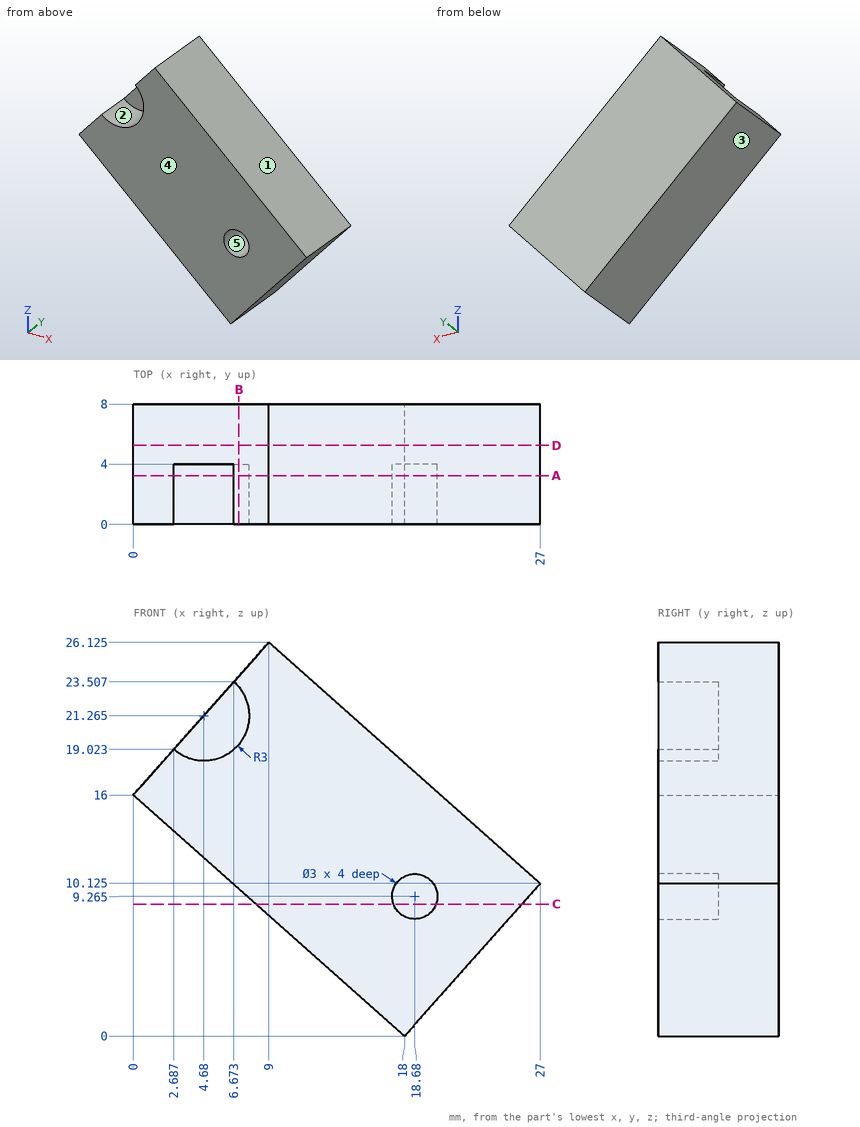
Study the drawing (mm; zero at the part's minimum x, y, z) and answer. A direction names the side the tool comes from. Round coordinates to 2 decimals unless told otherwise and drop trailing zeros. Write each loop counter-clockwise with the first axis right and the second up, starting at its lowest first coordinate (ties: lowest second). Pieces come first, ordered by that corner, then holes. Notation, with made-up numbers: (83, 41.5) - (93, 41.5) arc R22 ccw to (93, 55.5) - close; hole circle Ø10 at (56, 28.5). An arc over 180 degrees is marked (long way). Return JSON: item names as keys, results as strings. Group by question number.
Q1. The mould has two halves that part along X. Classify the marked faces 1, 2 and 3: released by +X, released by -X, zero draft, split by the parting line, or undercut.
Q2. The part is cut by section D-D on y = 5.25. Write down the section's boundary in (x, z) (3 decimals).
Q3. Find the intervals of material crossed by L1, parallel to X at y = 3.5, z = 8.5 (1 decimal); L2, parallel to Z at x = 15, y = 2.25; L3, parallel to X at y = 5.75, z = 12, in increasing order.
Q4. For the marked faces 4 and 5, determine the directions among +Z, -Z, +X, -X, +Y, -Y from which every point of the face is accessible in a straight line to the end or side of a thin tool.
Q5. Each of these flat-tipped pins is pushed along its axis until it touches: pin 1 Ø4 at (x, z) = (5, 22) entering from -Y; pin 2 Ø1.5 at (x, y) = (23.5, 6.5) entering from -Z; pin 3 Ø1 at (x, y) = (15.5, 4.5) entering from +Z. Where does it stop, or does it pass through?
Q6. The part is cut by section B-B on x = 7. Write down the section's boundary in (y, z) (1 decimal).
Q7. The part is cut by section C-C on z = 8.75. Write down the section's boundary in (x, y), then the cut area to 3 significant figures.
Q8. The part is cut by section A-A on y = 3.25. Write down the section's boundary in (x, z) (1 decimal).
Solved:
{
 "1": {"face 1": "released by +X", "face 2": "undercut", "face 3": "released by -X"},
 "2": {"outline": "(0, 16) - (18, 0) - (27, 10.125) - (9, 26.125) - close"},
 "3": {"L1": "8.4 to 17.4, 20 to 25.6", "L2": "2.67 to 20.79", "L3": "4.5 to 24.89"},
 "4": {"face 4": "+Z, -Z, +X, -X, -Y", "face 5": "-Y"},
 "5": {"pin 1": "y = 4", "pin 2": "z = 5.34", "pin 3": "z = 20.79"},
 "6": {"outline": "(0, 9.8) - (8, 9.8) - (8, 23.9) - (0, 23.9) - (0, 23.2) - (4, 23.2) - (4, 19.4) - (0, 19.4) - close"},
 "7": {"outline": "(8.16, 0) - (17.27, 0) - (17.27, 4) - (20.09, 4) - (20.09, 0) - (25.78, 0) - (25.78, 8) - (8.16, 8) - close", "area": "130 mm²"},
 "8": {"outline": "(0, 16) - (18, 0) - (27, 10.1) - (9, 26.1) - (6.7, 23.5) arc R3 cw to (2.7, 19) - close; hole circle Ø3 at (18.7, 9.3)"}
}
